Autodesk Fusion 360 part; units mm, degrees
sketch "Sketch1" plane through (0, 0, 0) normal (1, 0, 0) x (0, 1, 0)
  line L0 (0, 0) -> (100, 0)
  line L1 (100, 0) -> (100, 100)
  line L2 (100, 100) -> (0, 100)
  line L3 (0, 100) -> (0, 0)
  line L4 (50, 10) -> (80, 10)
  line L5 (50, 60) -> (20, 60)
  line L6 (20, 60) -> (80, 60)
  line L7 (80, 60) -> (80, 10)
  line L8 (80, 10) -> (20, 10)
  line L9 (20, 10) -> (20, 60)
  line L10 (35, 65) -> (65, 65)
  line L11 (65, 65) -> (65, 80)
  line L12 (65, 80) -> (35, 80)
  line L13 (35, 80) -> (35, 65)
  line L14 (50, 85) -> (63, 85)
  line L15 (50, 97) -> (37, 97)
  line L16 (37, 97) -> (63, 97)
  line L17 (63, 97) -> (63, 85)
  line L18 (63, 85) -> (37, 85)
  line L19 (37, 85) -> (37, 97)
  dimension "d1" = 100
  dimension "d2" = 100
  dimension "d4" = 30
  dimension "d5" = 13
  dimension "d6" = 12
  dimension "d7" = 13
extrude "Extrude1" add sketch "Sketch1" along normal blind 3
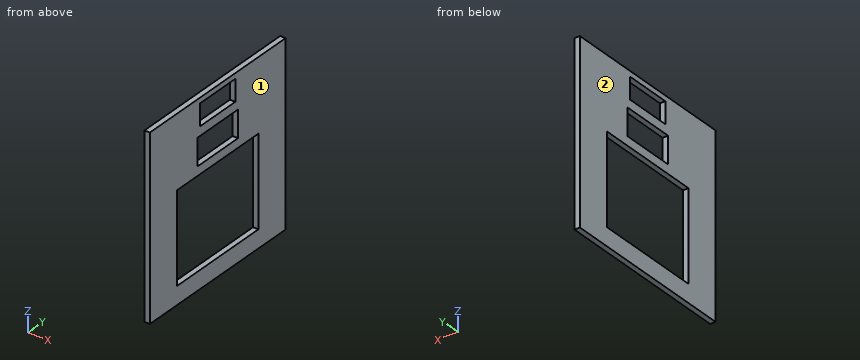
Could you check a few things on this model? Use its own coordinates, in mm. Face numbers are marked on the shaded views. Round coordinates to 2 decimals unless told otherwise and drop trailing zeros. Write each loop counter-clockwise with the first axis right and the second up, starting at its lowest first coordinate (ties: lowest second). Pieces come first, ordered by that corner, then holes. Notation, with made-up numbers: (60.25, -8) - (92.25, -8) arc R24 ccw to (92.25, 3) - close; hole circle Ø1 at (35.25, -21.5). An arc over 180 degrees is marked (long way). Put each result on its own line as item: value. Start each with the question number.
(1) I need wall thicknesses on probe 1 along Z at (x, y) = (1.65, 62.5); probe 2 along Y at (x, z) = (0.2, 17); probe 3 along Y at (x, z) = (2.8, 90). Which ranges of each line are inside material? Lowest first, please.
(2) I want a section at B-B, the plane z = 74. Please give me the cut outline in (x, y).
(3) I want a section at D-D, the plane z = 33. Please give me the cut outline in (x, y), plus the area to 3 significant figures.
(4) I want a section at A-A, the plane y = 40.5. Please give me the cut outline in (x, z).
(5) Thinking about a two-plate mould opening in X: for the marked faces 1 and 2, which applies, released by +X, released by -X, zero draft, split by the parting line, or undercut?
(6) I want a section at C-C, the plane x = 1.8. Please give me the cut outline in (y, z), plus the area to 3 significant figures.
Here are the results:
1. probe 1: z = 0 to 10, 60 to 65, 80 to 85, 97 to 100
1. probe 2: y = 0 to 20, 80 to 100
1. probe 3: y = 0 to 37, 63 to 100
2. outline: (0, 0) - (3, 0) - (3, 35) - (0, 35) - close; (0, 65) - (3, 65) - (3, 100) - (0, 100) - close
3. outline: (0, 0) - (3, 0) - (3, 20) - (0, 20) - close; (0, 80) - (3, 80) - (3, 100) - (0, 100) - close
3. area: 120 mm^2
4. outline: (0, 0) - (3, 0) - (3, 10) - (0, 10) - close; (0, 60) - (3, 60) - (3, 65) - (0, 65) - close; (0, 80) - (3, 80) - (3, 85) - (0, 85) - close; (0, 97) - (3, 97) - (3, 100) - (0, 100) - close
5. face 1: released by +X
5. face 2: released by -X
6. outline: (0, 0) - (100, 0) - (100, 100) - (0, 100) - close; hole (20, 10) - (80, 10) - (80, 60) - (20, 60) - close; hole (35, 65) - (65, 65) - (65, 80) - (35, 80) - close; hole (37, 85) - (63, 85) - (63, 97) - (37, 97) - close
6. area: 6,240 mm^2
